CAD build for the part. Positions are in the model's coordinates, mm. Face numbers are marked on the shaded views. A direction names the side the tool comes from. Give positions to 0.01 mm unless a question says otherwise; leave off trailing zeros. Order: outer loops, then holes, each group sorted by start corner. A loop starts at its lowest first (then second) coordinate and runs counter-clockwise, first axis right, second up.
Item 1: Wall check: L1, parallel to Y at x = 17.5, z = 0.3; L2, parallel to Z at x = -1, y = -9.75; L3, parallel to Z at x = 3, y = 6.25. Give the ranges that are in metal, low to high.
Item 2: Band-saw the part on B-B on x = 0. Give the cut face in (y, z), plus the area to 3 significant figures.
Item 3: Band-saw the part on D-D on y = -9.5. Give the cut face in (x, z).
Item 4: Band-saw the part on C-C on z = 11.5. Give the cut face in (x, y).
Item 5: Which spindle directions (+Z, -Z, +X, -X, +Y, -Y) get a long thin tool onto all of the face, cutting with end or side? Do the marked faces 1, 2, 3 and 4. Say none if no direction does.
Item 6: Flat gauge pins, fed straight in: P1, Ø15, axis at x = -8, y = -7.5, coming from the -Z side; P2, Ø7.5, axis at x = -18, y = 1.5, coming from the +Z side; P3, Ø7.5, axis at x = 15.5, y = 0, coming from the +Z side; P4, Ø0.5, axis at x = 14.5, z = 0.5, coming from the +Y side. Where does each tip first touch, or does it go through?
Item 7: Band-saw the part on A-A on y = 0. Give the cut face in (x, z), plus the area to 3 significant figures.
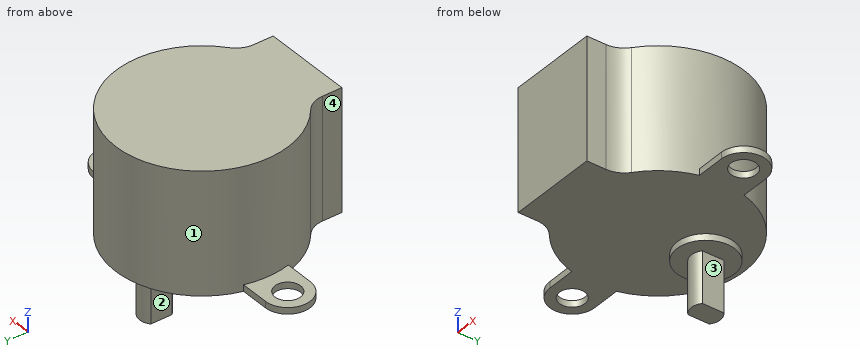
```python
from build123d import *

# Parameters (mm, degrees)
F1_DEPTH = 19
F2_R     = 2
F3_DEPTH = 1
F4_R     = 4.5
F5_DEPTH = 1
F7_DEPTH = 8


with BuildPart() as f1:
    # F0 (on Top) → F1 (new body)
    with BuildSketch(Plane.XY):
        with BuildLine():
            ThreePointArc((7, -13.5), (7.3731475524, -11.8648488215), (8.4187082405, -10.5534521158))
            ThreePointArc((8.4187082405, -10.5534521158), (0, 13.5), (-8.4187082405, -10.5534521158))
            ThreePointArc((-8.4187082405, -10.5534521158), (-7.3731475524, -11.8648488215), (-7, -13.5))
            Line((-7, -13.5), (-7, -16.5))
            Line((-7, -16.5), (7, -16.5))
            Line((7, -16.5), (7, -13.5))
        make_face()
    extrude(amount=F1_DEPTH)

    # F2 (on Top) → F3 (join)
    with BuildSketch(Plane.XY):
        with BuildLine():
            ThreePointArc((13.0384048104, 3.5), (13.5, 0), (13.0384048104, -3.5))
            Line((13.0384048104, -3.5), (17.5, -3.5))
            ThreePointArc((17.5, -3.5), (21, 0), (17.5, 3.5))
            Line((17.5, 3.5), (13.0384048104, 3.5))
        make_face()
        with Locations((17.5, 0)):
            Circle(F2_R, mode=Mode.SUBTRACT)
        with BuildLine():
            Line((-17.5, -3.5), (-13.0384048104, -3.5))
            ThreePointArc((-13.0384048104, -3.5), (-13.5, 0), (-13.0384048104, 3.5))
            Line((-13.0384048104, 3.5), (-17.5, 3.5))
            ThreePointArc((-17.5, 3.5), (-21, 0), (-17.5, -3.5))
        make_face()
        with Locations((-17.5, 0)):
            Circle(F2_R, mode=Mode.SUBTRACT)
    extrude(amount=F3_DEPTH)

    # F4 (on face) → F5 (join)
    with BuildSketch(Plane(origin=(0, 0, 0), x_dir=(1, 0, 0), z_dir=(0, 0, -1))):
        with Locations((0, -7.5)):
            Circle(F4_R)
    extrude(amount=F5_DEPTH)

    # F6 (on face) → F7 (join)
    with BuildSketch(Plane(origin=(0, 0, -1), x_dir=(1, 0, 0), z_dir=(0, 0, -1))):
        with BuildLine():
            Line((-1.5, -5.8229490169), (-1.5, -9.1770509831))
            ThreePointArc((-1.5, -9.1770509831), (0, -9.75), (1.5, -9.1770509831))
            Line((1.5, -9.1770509831), (1.5, -5.8229490169))
            ThreePointArc((1.5, -5.8229490169), (0, -5.25), (-1.5, -5.8229490169))
        make_face()
    extrude(amount=F7_DEPTH)


solid = f1.part
```
The answers:
1. L1: y = -3.5 to -2, 2 to 3.5
1. L2: z = 0 to 19
1. L3: z = -1 to 19
2. outline: (-16.5, 0) - (3, 0) - (3, -1) - (5.25, -1) - (5.25, -9) - (9.75, -9) - (9.75, -1) - (12, -1) - (12, 0) - (13.5, 0) - (13.5, 19) - (-16.5, 19) - close
2. area: 615 mm2
3. outline: (-9.59, 0) - (9.59, 0) - (9.59, 19) - (-9.59, 19) - close
4. outline: (-8.42, -10.55) arc R3.77 cw to (-7, -13.5) - (-7, -16.5) - (7, -16.5) - (7, -13.5) arc R3.77 cw to (8.42, -10.55) arc R13.5 ccw (long way) to start
5. face 1: +Z
5. face 2: -Z, -X, +Y, -Y
5. face 3: -Z, +X, +Y, -Y
5. face 4: +Z, -Z, -X, -Y
6. P1: stops at z = 0
6. P2: stops at z = 1
6. P3: stops at z = 19
6. P4: stops at y = 3.5
7. outline: (-21, 0) - (-19.5, 0) - (-19.5, 1) - (-21, 1) - close; (-15.5, 0) - (15.5, 0) - (15.5, 1) - (13.5, 1) - (13.5, 19) - (-13.5, 19) - (-13.5, 1) - (-15.5, 1) - close; (19.5, 0) - (21, 0) - (21, 1) - (19.5, 1) - close
7. area: 520 mm2
